The model under review builds one solid part; all positions refer to its coordinate system, in mm. Face numbers are marked on the shaded views. A direction names the side the tool comes from. Coordinates: 2 decimals unless noted, no trailing zeros. Loops run counter-clockwise (first coordinate to the right, second up) from the corner with the lowest first, then second, coordinate; pieces in that order, holes last. Notation, with made-up numbers: M 59.5,-29 L 79.5,-29 A17 cw 79.5,3 Z; hole C 85.25,-31.5 d11. An arc over 180 degrees is marked long. Return JSON: item names as keys, results as strings.
```python
from build123d import *

# Parameters (mm, degrees)
BOSS_EXTRUDE1_DEPTH = 17
SKETCH2_R           = 1.5
BOSS_EXTRUDE2_DEPTH = 5
SKETCH3_W           = 30
SKETCH3_H           = 7.1
SKETCH3_W_2         = 8.1
SKETCH3_H_2         = 2.2
CUT_EXTRUDE1_DEPTH  = 5
CHAMFER1_SIZE       = 2


with BuildPart() as part:
    # Sketch1 → Boss-Extrude1 (new, symmetric)
    with BuildSketch(Plane(origin=(0, 0, 0), x_dir=(0, 0, -1), z_dir=(1, 0, 0))):
        Polygon((0, 0), (50.5, 0), (50.5, 11.1), (14.5, 11.1), (12, 15.1), (0, 15.1), align=None)
    extrude(amount=BOSS_EXTRUDE1_DEPTH, both=True)

    # Sketch2 → Boss-Extrude2 (add)
    with BuildSketch(Plane(origin=(0, 0, -50.5), x_dir=(-1, 0, 0), z_dir=(0, 0, -1))):
        with Locations(Location((9.625, 5.55, 0), (0, 0, 180))):
            Circle(SKETCH2_R)
        with Locations(Location((-9.625, 5.55, 0), (0, 0, 180))):
            Circle(SKETCH2_R)
    extrude(amount=BOSS_EXTRUDE2_DEPTH)

    # Sketch3 → Cut-Extrude1 (cut)
    with BuildSketch(Plane.XY):
        with Locations((0, 5.55)):
            Rectangle(SKETCH3_W, SKETCH3_H)
        with Locations((-4.55, 12)):
            Rectangle(SKETCH3_W_2, SKETCH3_H_2)
        with Locations((4.55, 12)):
            Rectangle(SKETCH3_W_2, SKETCH3_H_2)
    extrude(amount=-CUT_EXTRUDE1_DEPTH, mode=Mode.SUBTRACT)

    # Chamfer1
    chamfer1_edges = [part.edges().sort_by_distance(p)[0] for p in [
        (0, 11.1, -50.5),
        (0, 0, -50.5),
        (17, 5.55, -50.5),
        (17, 11.1, -32.5),
        (17, 13.1, -13.25),
        (17, 15.1, -6),
        (-17, 15.1, -6),
        (-17, 13.1, -13.25),
        (-17, 11.1, -32.5),
        (-17, 5.55, -50.5),
        (-17, 0, -25.25),
        (17, 0, -25.25),
    ]]
    chamfer(chamfer1_edges, length=CHAMFER1_SIZE)


solid = part.part
```
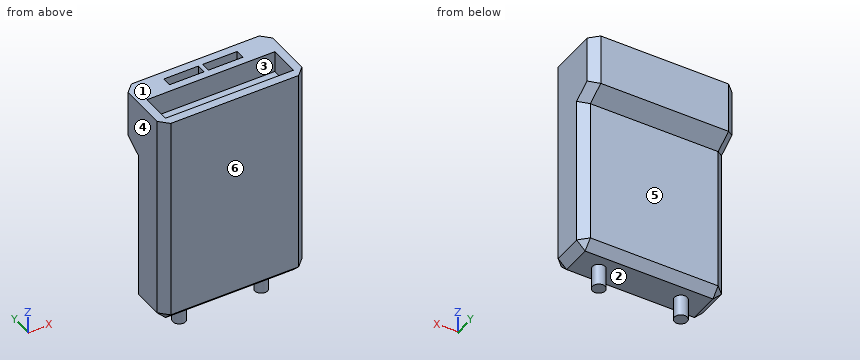
1. Add section B-B on y = 5.55. Give the boundary of the cut face in (x, z) (3 decimals), plus the area to 3 significant figures.
Check values:
{"outline": "M -17,-48.5 L -15,-50.5 L -11.125,-50.5 L -11.125,-55.5 L -8.125,-55.5 L -8.125,-50.5 L 8.125,-50.5 L 8.125,-55.5 L 11.125,-55.5 L 11.125,-50.5 L 15,-50.5 L 17,-48.5 L 17,0 L 15,0 L 15,-5 L -15,-5 L -15,0 L -17,0 Z", "area": "1,590 mm²"}
2. To check wall thickness, follow line 1 (X direction, y = 3.75, z = -4.5); line 2 (Y direction, x = 5.5, z = -44); line 3 (Z direction, x = 14, y = 8.5). State the ranges of each line that lie inside material, in increasing order.
Check values:
{"line 1": "-17 to -15, 15 to 17", "line 2": "0 to 11.1", "line 3": "-50.5 to -5"}
3. Add section A-A on z = -20.5. Give the boundary of the cut face in (x, y).
Check values:
{"outline": "M -17,2 L -15,0 L 15,0 L 17,2 L 17,9.1 L 15,11.1 L -15,11.1 L -17,9.1 Z"}
4. The part is to be moulded in two halves that separate along X. For the marked faces 1, 2, 3 and 4, say which applies: released by +X, released by -X, zero draft, split by the parting line, or undercut.
Check values:
{"face 1": "zero draft", "face 2": "undercut", "face 3": "undercut", "face 4": "released by -X"}
5. Add section C-C on z = -6. Give the boundary of the cut face in (x, y), plus the area to 3 significant figures.
Check values:
{"outline": "M -17,2 L -15,0 L 15,0 L 17,2 L 17,13.1 L 15,15.1 L -15,15.1 L -17,13.1 Z", "area": "505 mm²"}
6. Machinability: for the marked faces 5 and 6, which of the approach directions +Z, -Z, +X, -X, +Y, -Y give a long, thin tool a straight path to every point of the face, cutting with its end or side? Answer none if there is none.
Check values:
{"face 5": "-Z, +X, -X, +Y", "face 6": "+Z, -Z, +X, -X, -Y"}
7. Insertion check: pin 1 Ø3 at (y, z) = (10, -35) entering from -X; pin 2 Ø5.5 at (x, y) = (0.5, 6) entering from -Z; pin 3 Ø10 at (x, z) = (-13, -19) entering from +Y; pin 4 Ø1.1 at (x, y) = (-3.5, 11.5) entering from +Z. Each pin has a flat end and moves straight along its axis. Give the tip position at first contact, or say it passes through.
Check values:
{"pin 1": "x = -17", "pin 2": "z = -50.5", "pin 3": "y = 11.9", "pin 4": "z = -5"}
